from build123d import *

# Parameters (mm, degrees)
SKETCH1_W           = 300
SKETCH1_H           = 300
BOSS_EXTRUDE1_DEPTH = 3
SKETCH2_W           = 16
SKETCH2_H           = 100
CUT_EXTRUDE2_DEPTH  = 3
SKETCH3_W           = 16
SKETCH3_H           = 100
CUT_EXTRUDE3_DEPTH  = 3
SKETCH5_W           = 40
SKETCH5_H           = 60
CUT_EXTRUDE4_DEPTH  = 3
SKETCH6_R           = 2.5
CUT_EXTRUDE5_DEPTH  = 3
CUT_EXTRUDE6_DEPTH  = 3
CUT_EXTRUDE7_DEPTH  = 3


with BuildPart() as part:
    # Sketch1 → Boss-Extrude1 (new body)
    with BuildSketch(Plane(origin=(0, 0, 0), x_dir=(1, 0, 0), z_dir=(0, 1, 0))):
        Rectangle(SKETCH1_W, SKETCH1_H)
    extrude(amount=BOSS_EXTRUDE1_DEPTH)

    # Sketch2 → Cut-Extrude2 (cut)
    with BuildSketch(Plane(origin=(0, 3, 0), x_dir=(1, 0, 0), z_dir=(0, 1, 0))):
        with Locations((-106.999981758, -49.997456266)):
            Rectangle(SKETCH2_W, SKETCH2_H)
    extrude(amount=-CUT_EXTRUDE2_DEPTH, mode=Mode.SUBTRACT)

    # Sketch3 → Cut-Extrude3 (cut)
    with BuildSketch(Plane(origin=(0, 3, 0), x_dir=(1, 0, 0), z_dir=(0, 1, 0))):
        with Locations((106.997905593, -50.002067411)):
            Rectangle(SKETCH3_W, SKETCH3_H)
    extrude(amount=-CUT_EXTRUDE3_DEPTH, mode=Mode.SUBTRACT)

    # Sketch5 → Cut-Extrude4 (cut)
    with BuildSketch(Plane(origin=(0, 3, 0), x_dir=(1, 0, 0), z_dir=(0, 1, 0))):
        with Locations((0.000226616, 103.221805272)):
            Rectangle(SKETCH5_W, SKETCH5_H)
    extrude(amount=-CUT_EXTRUDE4_DEPTH, mode=Mode.SUBTRACT)

    # Sketch6 → Cut-Extrude5 (cut)
    with BuildSketch(Plane(origin=(0, 3, 0), x_dir=(1, 0, 0), z_dir=(0, 1, 0))):
        with Locations((-126.465787007, -29.019127059)):
            Circle(SKETCH6_R)
        with Locations((-86.465787007, -29.019127059)):
            Circle(SKETCH6_R)
        with Locations((-126.465787007, -71.019127059)):
            Circle(SKETCH6_R)
        with Locations((-86.465787007, -71.019127059)):
            Circle(SKETCH6_R)
        with Locations((86.681368776, -29.075116819)):
            Circle(SKETCH6_R)
        with Locations((86.681368776, -71.075116819)):
            Circle(SKETCH6_R)
        with Locations((126.681368776, -29.075116819)):
            Circle(SKETCH6_R)
        with Locations((126.681368776, -71.075116819)):
            Circle(SKETCH6_R)
        with Locations((-25, 118)):
            Circle(SKETCH6_R)
        with Locations((-25, 88)):
            Circle(SKETCH6_R)
        with Locations((25, 118)):
            Circle(SKETCH6_R)
        with Locations((25, 88)):
            Circle(SKETCH6_R)
    extrude(amount=-CUT_EXTRUDE5_DEPTH, mode=Mode.SUBTRACT)

    # Sketch7 → Cut-Extrude6 (cut)
    with BuildSketch(Plane(origin=(0, 3, 0), x_dir=(1, 0, 0), z_dir=(0, 1, 0))):
        with BuildLine():
            Line((-104.3, 52.5), (-104.3, 37.5))
            ThreePointArc((-104.3, 37.5), (-106, 35.8), (-107.7, 37.5))
            Line((-107.7, 37.5), (-107.7, 52.5))
            ThreePointArc((-107.7, 52.5), (-106, 54.2), (-104.3, 52.5))
        make_face()
        with BuildLine():
            Line((-104.3, 32.5), (-104.3, 17.5))
            ThreePointArc((-104.3, 17.5), (-106, 15.8), (-107.7, 17.5))
            Line((-107.7, 17.5), (-107.7, 32.5))
            ThreePointArc((-107.7, 32.5), (-106, 34.2), (-104.3, 32.5))
        make_face()
        with BuildLine():
            Line((-80.3, 52.5), (-80.3, 37.5))
            ThreePointArc((-80.3, 37.5), (-82, 35.8), (-83.7, 37.5))
            Line((-83.7, 37.5), (-83.7, 52.5))
            ThreePointArc((-83.7, 52.5), (-82, 54.2), (-80.3, 52.5))
        make_face()
        with BuildLine():
            Line((-80.3, 32.5), (-80.3, 17.5))
            ThreePointArc((-80.3, 17.5), (-82, 15.8), (-83.7, 17.5))
            Line((-83.7, 17.5), (-83.7, 32.5))
            ThreePointArc((-83.7, 32.5), (-82, 34.2), (-80.3, 32.5))
        make_face()
        with BuildLine():
            Line((83.7, 52.5), (83.7, 37.5))
            ThreePointArc((83.7, 37.5), (82, 35.8), (80.3, 37.5))
            Line((80.3, 37.5), (80.3, 52.5))
            ThreePointArc((80.3, 52.5), (82, 54.2), (83.7, 52.5))
        make_face()
        with BuildLine():
            Line((83.7, 32.5), (83.7, 17.5))
            ThreePointArc((83.7, 17.5), (82, 15.8), (80.3, 17.5))
            Line((80.3, 17.5), (80.3, 32.5))
            ThreePointArc((80.3, 32.5), (82, 34.2), (83.7, 32.5))
        make_face()
        with BuildLine():
            Line((107.7, 52.5), (107.7, 37.5))
            ThreePointArc((107.7, 37.5), (106, 35.8), (104.3, 37.5))
            Line((104.3, 37.5), (104.3, 52.5))
            ThreePointArc((104.3, 52.5), (106, 54.2), (107.7, 52.5))
        make_face()
        with BuildLine():
            Line((107.7, 32.5), (107.7, 17.5))
            ThreePointArc((107.7, 17.5), (106, 15.8), (104.3, 17.5))
            Line((104.3, 17.5), (104.3, 32.5))
            ThreePointArc((104.3, 32.5), (106, 34.2), (107.7, 32.5))
        make_face()
    extrude(amount=-CUT_EXTRUDE6_DEPTH, mode=Mode.SUBTRACT)

    # Sketch8 → Cut-Extrude7 (cut)
    with BuildSketch(Plane(origin=(0, 3, 0), x_dir=(1, 0, 0), z_dir=(0, 1, 0))):
        with BuildLine():
            Line((-99, -105.5), (-99, -120.5))
            ThreePointArc((-99, -120.5), (-100, -121.5), (-101, -120.5))
            Line((-101, -120.5), (-101, -105.5))
            ThreePointArc((-101, -105.5), (-100, -104.5), (-99, -105.5))
        make_face()
        with BuildLine():
            Line((-99, -127.5), (-99, -142.5))
            ThreePointArc((-99, -142.5), (-100, -143.5), (-101, -142.5))
            Line((-101, -142.5), (-101, -127.5))
            ThreePointArc((-101, -127.5), (-100, -126.5), (-99, -127.5))
        make_face()
        with BuildLine():
            Line((101, -105.5), (101, -120.5))
            ThreePointArc((101, -120.5), (100, -121.5), (99, -120.5))
            Line((99, -120.5), (99, -105.5))
            ThreePointArc((99, -105.5), (100, -104.5), (101, -105.5))
        make_face()
        with BuildLine():
            Line((101, -127.5), (101, -142.5))
            ThreePointArc((101, -142.5), (100, -143.5), (99, -142.5))
            Line((99, -142.5), (99, -127.5))
            ThreePointArc((99, -127.5), (100, -126.5), (101, -127.5))
        make_face()
    extrude(amount=-CUT_EXTRUDE7_DEPTH, mode=Mode.SUBTRACT)


solid = part.part
Could you check a few things on this model? Use its own coordinates, in mm. Give positions to 0.01 mm unless a question says otherwise; leave off trailing zeros. Order: outer loops, then holes, each group sorted by start corner. A loop starts at its lowest first (then second) coordinate and runs counter-clockwise, first axis right, second up. Notation, with made-up numbers: (87.5, 74.25) - (112.5, 74.25) arc R26 ccw to (112.5, 108.25) - close; hole circle Ø4 at (-10, 54.25). An arc over 180 degrees is marked (long way). Return JSON: item names as keys, results as strings. Group by question number.
Q1. Will this pin go through, and if not, where does the flat tip stop? pin 1 Ø4 at (x, z) = (-25, -118) entering from -Y.
Q2. Please list where these lines run through material, in increasing order: line 1 along X through (y, z) = (0.65, -41.5); line 2 along Z through (x, y) = (-25, 1.75); line 3 along X through (y, z) = (1.65, -118). Write a range as [from, to].
Q3. Suppose I cut it at B-B, the plane y = 2.45. State how many separate pieces and enclosed holes the cut face has, and give its area (3 significant figures).
Q4. Suppose I cut it at A-A, the plane z = -103.5. Please give me the cut outline in (x, y), and give its area (3 significant figures).
Resolved:
{
 "1": {"pin 1": "passes through"},
 "2": {"line 1": "x = [-150, -107.7], [-104.3, -83.7], [-80.3, 80.3], [83.7, 104.3], [107.7, 150]", "line 2": "z = [-150, -120.5], [-115.5, -90.5], [-85.5, 150]", "line 3": "x = [-150, -27.5], [-22.5, -20], [20, 22.5], [27.5, 150]"},
 "3": {"separate pieces": "1", "enclosed holes": "27", "area": "83,600 mm2"},
 "4": {"outline": "(-150, 0) - (-20, 0) - (-20, 3) - (-150, 3) - close; (20, 0) - (150, 0) - (150, 3) - (20, 3) - close", "area": "780 mm2"}
}
